from build123d import *

# Parameters (mm, degrees)
SKETCH1_W           = 13.25
SKETCH1_H           = 110.001600164
BOSS_EXTRUDE1_DEPTH = 1.6002
SKETCH2_R           = 2.0574
CUT_EXTRUDE1_DEPTH  = 111.808281183
SKETCH3_R           = 5.699999998
CUT_EXTRUDE2_DEPTH  = 111.808281183


with BuildPart() as part:
    # Sketch1 → Boss-Extrude1 (new body)
    with BuildSketch(Plane(origin=(0, 0, 0), x_dir=(1, 0, 0), z_dir=(0, 1, 0))):
        with Locations((6.625, 55.000800082)):
            Rectangle(SKETCH1_W, SKETCH1_H)
    extrude(amount=BOSS_EXTRUDE1_DEPTH)

    # Sketch2 → Cut-Extrude1 (cut, through all)
    with BuildSketch(Plane(origin=(0, 1.6002, 0), x_dir=(1, 0, 0), z_dir=(0, 1, 0))):
        with Locations(Location((6.625, 4.7244, 0), (0, 0, 270))):
            Circle(SKETCH2_R)
        with Locations(Location((6.625, 105.277200164, 0), (0, 0, 270))):
            Circle(SKETCH2_R)
    extrude(amount=-CUT_EXTRUDE1_DEPTH, mode=Mode.SUBTRACT)

    # Sketch3 → Cut-Extrude2 (cut, through all)
    with BuildSketch(Plane(origin=(0, 1.6002, 0), x_dir=(1, 0, 0), z_dir=(0, 1, 0))):
        with Locations((-4.699999998, 88.909788652)):
            Circle(SKETCH3_R)
        with Locations((-4.699999998, 66.303788652)):
            Circle(SKETCH3_R)
        with Locations((-4.699999998, 43.697788652)):
            Circle(SKETCH3_R)
        with Locations((-4.699999998, 21.091788652)):
            Circle(SKETCH3_R)
        with Locations((17.949999998, 21.091788652)):
            Circle(SKETCH3_R)
        with Locations((17.949999998, 43.697788652)):
            Circle(SKETCH3_R)
        with Locations((17.949999998, 66.303788652)):
            Circle(SKETCH3_R)
        with Locations((17.949999998, 88.909788652)):
            Circle(SKETCH3_R)
    extrude(amount=-CUT_EXTRUDE2_DEPTH, mode=Mode.SUBTRACT)


solid = part.part
Geometry check sheet. Reference: the model listing, model coordinates, mm. Give positions to 0.01 mm unless a question says otherwise; leave off trailing zeros. Order: outer loops, then holes, each group sorted by start corner. A loop starts at its lowest first (then second) coordinate and runs counter-clockwise, first axis right, second up.
1) Cross-section at A-A (y = 0.6). Record the boundary of the cut face in (x, z) (3 decimals).
Results are:
outline: (0, -110.002) - (13.25, -110.002) - (13.25, -92.135) arc R5.7 cw to (13.25, -85.685) - (13.25, -69.529) arc R5.7 cw to (13.25, -63.079) - (13.25, -46.923) arc R5.7 cw to (13.25, -40.473) - (13.25, -24.317) arc R5.7 cw to (13.25, -17.867) - (13.25, 0) - (0, 0) - (0, -17.867) arc R5.7 cw to (0, -24.317) - (0, -40.473) arc R5.7 cw to (0, -46.923) - (0, -63.079) arc R5.7 cw to (0, -69.529) - (0, -85.685) arc R5.7 cw to (0, -92.135) - close; hole circle Ø4.115 at (6.625, -105.277); hole circle Ø4.115 at (6.625, -4.724)
2) Draft check along X on faces 1 (the cylindrical face through (8.015, 0.811, -6.241)), 2 (the flat face through (7, 0, -56)). Enter one of: released by +X, released by -X, zero draft, split by the parting line, or undercut.
Results are:
face 1: undercut
face 2: zero draft
3) Material ranges on probe 1 along Z at (x, y) = (0.5, 1.5); probe 2 along Z at (x, y) = (7, 1.15); probe 3 along Z at (x, y) = (5.25, 0.5), recorded low to high.
Results are:
probe 1: z = -110 to -91.24, -86.58 to -68.64, -63.97 to -46.03, -41.36 to -23.43, -18.76 to 0
probe 2: z = -110 to -107.3, -103.25 to -6.75, -2.7 to 0
probe 3: z = -110 to -106.81, -103.75 to -6.25, -3.19 to 0
4) Cross-section at B-B (z = -42). Record the boundary of the cut face in (x, y), then the cut area to 3 significant figures.
Results are:
outline: (0.74, 0) - (12.51, 0) - (12.51, 1.6) - (0.74, 1.6) - close
area: 18.8 mm2
